from build123d import *

# Parameters (mm, degrees)
F1_DEPTH      = 384.302
F3_DEPTH      = 25.4
F3_DEPTH_BACK = 25.4


with BuildPart() as f1:
    # F0 (on Right) → F1 (new body)
    with BuildSketch(Plane.YZ):
        with BuildLine():
            ThreePointArc((25.4, 22.225), (24.4700640303, 24.4700640303), (22.225, 25.4))
            Line((22.225, 25.4), (-22.225, 25.4))
            ThreePointArc((-22.225, 25.4), (-24.4700640303, 24.4700640303), (-25.4, 22.225))
            Line((-25.4, 22.225), (-25.4, -22.225))
            ThreePointArc((-25.4, -22.225), (-24.4700640303, -24.4700640303), (-22.225, -25.4))
            Line((-22.225, -25.4), (22.225, -25.4))
            ThreePointArc((22.225, -25.4), (24.4700640303, -24.4700640303), (25.4, -22.225))
            Line((25.4, -22.225), (25.4, 22.225))
        make_face()
        with BuildLine():
            Line((-19.05, 22.225), (19.05, 22.225))
            ThreePointArc((19.05, 22.225), (21.2950640303, 21.2950640303), (22.225, 19.05))
            Line((22.225, 19.05), (22.225, -19.05))
            ThreePointArc((22.225, -19.05), (21.2950640303, -21.2950640303), (19.05, -22.225))
            Line((19.05, -22.225), (-19.05, -22.225))
            ThreePointArc((-19.05, -22.225), (-21.2950640303, -21.2950640303), (-22.225, -19.05))
            Line((-22.225, -19.05), (-22.225, 19.05))
            ThreePointArc((-22.225, 19.05), (-21.2950640303, 21.2950640303), (-19.05, 22.225))
        make_face(mode=Mode.SUBTRACT)
    extrude(amount=F1_DEPTH)

    # F2 (on Front) → F3 (cut, two sides)
    with BuildSketch(Plane.XZ) as f3_sk:
        Polygon((0, -25.4), (50.8, -25.4), (0, 25.4), align=None)
    extrude(amount=-F3_DEPTH, mode=Mode.SUBTRACT)
    extrude(f3_sk.sketch, amount=F3_DEPTH_BACK, mode=Mode.SUBTRACT)


solid = f1.part
Check sheet for the modelled part. Datum: model origin and axes. Units: mm. A direction names the side the tool comes from. Round coordinates to 2 decimals unless told otherwise and drop trailing zeros. Order: outer loops, then holes, each group sorted by start corner. A loop starts at its lowest first (then second) coordinate and runs counter-clockwise, first axis right, second up. Notation, with made-up numbers: M 89,20.5 L 138,20.5 A9 ccw 138,32.5 Z; hole C 40,33 d8. An arc over 180 degrees is marked long. One line per item, written item: value. Start each with the question number.
1. Section check B-B on z = -5.5. Enter the section's corners in (x, y) (3 decimals), and give its area (3 significant figures).
2. Section check A-A on y = -5.5. Enter the section's corners in (x, z) (3 decimals).
3. Release check for a two-part mould opening along Z. For faces 3 (the flat face through (191, -25.4, 0)), 4 (the flat face through (23.6, 22.5, 1.8)), 5 (the flat face through (191, 0, 22.225)) record: released by +Z, released by -Z, zero draft, split by the parting line, or undercut.
4. Access from +Z, -Z, +X, -X, +Y, -Y to the whole of each face (thin tool, end or side, straight path). Record for faces 1 (the flat face through (215, 0, -25.4)), 2 (the flat face through (214, 0, -22.225)).
5. Scan lines: line 1 along Z through (x, y) = (364.5, 7.5) (3 decimals); line 2 along Z through (x, y) = (18.5, 2) (3 decimals). Record each from-to range of solid material in increasing order.
6. Section check C-C on x = 196.5. Enter the section's corners in (y, z) (3 decimals).
7. Gauge pin test, flat end, axial feed: P1, Ø12, axis at y = 10.5, z = 18, coming from the -X side. Record the tip position at first contact, or that the pin passes through.
Results found:
1. outline: M 30.9,-25.4 L 384.302,-25.4 L 384.302,-22.225 L 30.9,-22.225 Z; M 30.9,22.225 L 384.302,22.225 L 384.302,25.4 L 30.9,25.4 Z
1. area: 2,240 mm^2
2. outline: M 0,25.4 L 3.175,22.225 L 384.302,22.225 L 384.302,25.4 Z; M 47.625,-22.225 L 50.8,-25.4 L 384.302,-25.4 L 384.302,-22.225 Z
3. face 3: zero draft
3. face 4: released by -Z
3. face 5: undercut
4. face 1: -Z, +X, -X, +Y, -Y
4. face 2: +X, -X
5. line 1: -25.4 to -22.225, 22.225 to 25.4
5. line 2: 22.225 to 25.4
6. outline: M -25.4,-22.225 A3.175 ccw -22.225,-25.4 L 22.225,-25.4 A3.175 ccw 25.4,-22.225 L 25.4,22.225 A3.175 ccw 22.225,25.4 L -22.225,25.4 A3.175 ccw -25.4,22.225 Z; hole M -22.225,-19.05 A3.175 ccw -19.05,-22.225 L 19.05,-22.225 A3.175 ccw 22.225,-19.05 L 22.225,19.05 A3.175 ccw 19.05,22.225 L -19.05,22.225 A3.175 ccw -22.225,19.05 Z
7. P1: x = 1.4
